Autodesk Fusion 360 part; units mm, degrees
sketch "スケッチ1" plane through (0, 0, 0) normal (0, 0, 1) x (1, 0, 0)
  line L0 (0, 0) -> (-50, 0)
  line L1 (-50, 0) -> (-50, -35)
  line L2 (-50, -35) -> (0, -35)
  line L3 (0, -35) -> (0, 0)
  line L4 (-65, 5) -> (15, 5)
  line L5 (15, 5) -> (15, -40)
  line L6 (15, -40) -> (-65, -40)
  line L7 (-65, -40) -> (-65, 5)
extrude "押し出し1" add sketch "スケッチ1" against normal blind 5 contours L0 L1 L2 L3
extrude "押し出し2" add sketch "スケッチ1" along normal blind 5 contours L0 L1 L2 L3 | L4 L5 L6 L7
sketch "スケッチ2" plane through (0, 0, 5) normal (0, 0, 1) x (-1, 0, 0)
  line L0 (65, 40) -> (-15, 40)
  line L1 (-15, 40) -> (-15, -5)
  line L2 (-15, -5) -> (65, -5)
  line L3 (65, -5) -> (65, 40)
  line L4 (-15, 0) -> (65, 0)
  line L5 (65, 0) -> (65, 30)
  line L6 (65, 30) -> (-15, 30)
  line L7 (-15, 30) -> (-15, 0)
extrude "押し出し3" cut sketch "スケッチ2" against normal blind 3 contours L1 L3 L4 L5 L6 L7
sketch "スケッチ3" plane through (0, 0, -5) normal (0, 0, -1) x (1, 0, 0)
  line L0 (0, 0) -> (0, 35)
  line L1 (0, 35) -> (-50, 35)
  line L2 (-50, 35) -> (-50, 0)
  line L3 (-50, 0) -> (0, 0)
  line L4 (-10, 0) -> (-40, 0)
  line L5 (-40, 0) -> (-40, 35)
  line L6 (-40, 35) -> (-10, 35)
  line L7 (-10, 35) -> (-10, 0)
extrude "押し出し4" cut sketch "スケッチ3" against normal blind 10 contours L1 L3 L4 L5 L6 L7
extrude "押し出し5" add 2 faces at (-38.3333, 3.3333, 5) (-56.6667, -35, 5) along direction (0, 0, 1) blind 3
sketch "スケッチ4" plane through (-65, 0, 0) normal (-1, 0, 0) x (0, -1, 0)
  line L0 (0, 2) -> (0, 8)
  line L1 (0, 8) -> (-5, 8)
  line L2 (-5, 8) -> (-5, 0)
  line L3 (-5, 0) -> (40, 0)
  line L4 (40, 0) -> (40, 8)
  line L5 (40, 8) -> (30, 8)
  line L6 (30, 8) -> (30, 2)
  line L7 (30, 2) -> (0, 2)
  line L8 (0, 5) -> (30, 5)
  line L9 (0, 4) -> (30, 4)
  arc A0 (30, 4) -> (30, 6) centre (30, 5) ccw
  line L10 (30, 6) -> (0, 6)
  arc A1 (0, 6) -> (0, 4) centre (0, 5) ccw
  line L11 (0, 5) -> (30, 5) construction
extrude "押し出し6" cut sketch "スケッチ4" against normal blind 80 contours L0 A1 | L6 A0
sketch "スケッチ5" plane through (0, 0, -5) normal (0, 0, -1) x (1, 0, 0)
  line L0 (-40, 0) -> (-40, 35)
  line L1 (-40, 35) -> (-50, 35)
  line L2 (-50, 35) -> (-50, 0)
  line L3 (-50, 0) -> (-40, 0)
extrude "押し出し7" cut 1 faces at (-65, -36.9916, 4.2592) along direction (1, 0, 0) blind 1
extrude "押し出し8" cut 1 faces at (-64, -36.9916, 4.2592) along direction (1, 0, 0) blind 1
extrude "押し出し9" cut 1 faces at (15, -36.9916, 4.2592) along direction (-1, 0, 0) blind 1
extrude "押し出し10" add 1 faces at (-63, -36.9916, 4.2592) along direction (-1, 0, 0) blind 0.5
extrude "押し出し11" cut 1 faces at (14, -36.9916, 4.2592) along direction (-1, 0, 0) blind 0.5
extrude "押し出し12" cut 1 faces at (0, -23.3333, -3.3333) along direction (-1, 0, 0) blind 0.25
extrude "押し出し13" cut 1 faces at (-50, -11.6667, -3.3333) along direction (1, 0, 0) blind 0.25
extrude "押し出し14" add 1 faces at (-63.5, -36.9916, 4.2592) along direction (-1, 0, 0) blind 1
For this review, take the finished solid that the model builds, in its own axes (mm). A direction names the side the tool comes from. Coordinates: 2 decimals unless noted, no trailing zeros. Write each loop counter-clockwise with the first axis right and the second up, starting at its lowest first coordinate (ties: lowest second). Pieces come first, ordered by that corner, then holes. Notation, with made-up numbers: (13, -5) - (17, -5) arc R21 cw to (17, 16) - close; hole circle Ø6 at (-1.75, 89). An arc over 180 degrees is marked (long way). Put each result on its own line as item: value.
1. Mouldability with a two-part tool opening along X and no side actions: class faces 5 (the flat face through (-40, -17, -1)), 6 (the flat face through (-45, -17, -5)), 7 (the flat face through (13.5, -22, 1)) as released by +X, released by -X, zero draft, split by the parting line, or undercut.
Values found:
face 5: undercut
face 6: zero draft
face 7: released by +X
2. Add section B-B, the plane x = -19.5. Give the boundary of the cut face in (y, z), then the cut area to 3 significant figures.
Values found:
outline: (-40, 0) - (-35, 0) - (-35, 8) - (-40, 8) - close; (0, 0) - (5, 0) - (5, 8) - (0, 8) - (0, 6) arc R1 cw to (0, 4) - close
area: 78.4 mm²
3. Add section A-A, the plane z = -3.25. Give the boundary of the cut face in (x, y).
Values found:
outline: (-49.75, -35) - (-40, -35) - (-40, 0) - (-49.75, 0) - close; (-10, -35) - (-0.25, -35) - (-0.25, 0) - (-10, 0) - close
4. Add section C-C, the plane y = -28. Give the boundary of the cut face in (x, z).
Values found:
outline: (-64.5, 0) - (-49.75, 0) - (-49.75, -5) - (-40, -5) - (-40, 2) - (-64.5, 2) - close; (-10, -5) - (-0.25, -5) - (-0.25, 0) - (13.5, 0) - (13.5, 2) - (-10, 2) - close
5. Wall thickness on probe 1 along X at (y, z) = (-28, -3.5); probe 2 along X at (y, z) = (-24, 1); probe 3 along Z at (x, y) = (4.5, 2.5): over which ranges is each line inside the solid? List them lowest first.
Values found:
probe 1: -49.75 to -40, -10 to -0.25
probe 2: -64.5 to -40, -10 to 13.5
probe 3: 0 to 8
6. For pin 1 (3 mm diameter, centred on x = -7, y = -8, fed in from +Z); pin 2 (1.5 mm diameter, centred on y = -15, z = -3, fed in from -X); pin 3 (22.5 mm diameter, centred on x = -21.5, y = -21, fed in from -Z); pin 4 (5.5 mm diameter, centred on x = -4.5, z = -3, fed in from +Y), all flat-tipped, find the tip position at first contact; note any pin that passes through.
Values found:
pin 1: z = 2
pin 2: x = -49.75
pin 3: through
pin 4: y = 0
7. Add section D-D, the plane z = 5. Give the boundary of the cut face in (x, y).
Values found:
outline: (-64.5, -40) - (13.5, -40) - (13.5, -31) - (-10, -31) - (-10, -35) - (-40, -35) - (-40, -31) - (-64.5, -31) - close; (-64.5, 1) - (13.5, 1) - (13.5, 5) - (-64.5, 5) - close
8. Machinability: for faces 1 (the flat face through (-25, -35, 4)), 2 (the flat face through (-0.25, -18, -2)), 3 (the flat face through (-5, 0, -2)), 4 (the flat face through (-52, -30, 7)), which of the approach directions +Z, -Z, +X, -X, +Y, -Y give a long, thin tool a straight path to every point of the face, cutting with its end or side? Answer none if there is none.
Values found:
face 1: +Z, -Z
face 2: -Z, +X, +Y, -Y
face 3: -Z, +X, -X, +Y
face 4: +Z, +X, -X
